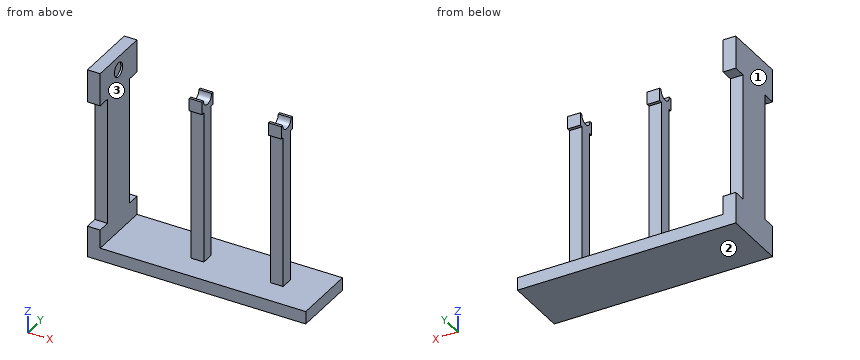
```python
from build123d import *

# Parameters (mm, degrees)
F0_W      = 411.1625
F0_H      = 127
F1_DEPTH  = 25.4
F2_W      = 25.4
F2_H      = 25.4
F3_DEPTH  = 304.8
F4_W      = 25.4
F4_H      = 38.1
F5_DEPTH  = 25.4
F7_DEPTH  = 258.7635
F8_W      = 127
F8_H      = 382.02858
F9_DEPTH  = 25.4
F10_W     = 89.525855
F10_H     = 254
F11_DEPTH = 25.4
F12_R     = 14.2875
F13_DEPTH = 340.36


with BuildPart() as f1:
    # F0 (on Top) → F1 (new body)
    with BuildSketch(Plane.XY):
        with Locations((0, 6.35)):
            Rectangle(F0_W, F0_H)
    extrude(amount=F1_DEPTH)

    # F2 (on face) → F3 (join)
    with BuildSketch(Plane.XY.offset(25.4)):
        with Locations((-40.48125, 6.35)):
            Rectangle(F2_W, F2_H)
        with Locations((118.26875, 6.35)):
            Rectangle(F2_W, F2_H)
    extrude(amount=F3_DEPTH)

    # F4 (on face) → F5 (join)
    with BuildSketch(Plane.XY.offset(330.2)):
        with Locations((-40.48125, 6.35)):
            Rectangle(F4_W, F4_H)
        with Locations((118.26875, 6.35)):
            Rectangle(F4_W, F4_H)
    extrude(amount=F5_DEPTH)

    # F6 (on face) → F7 (cut, through all)
    with BuildSketch(Plane(origin=(-53.18125, 0, 0), x_dir=(0, -1, 0), z_dir=(-1, 0, 0))):
        with BuildLine():
            Line((7.9375, 355.6), (-20.6375, 355.6))
            ThreePointArc((-20.6375, 355.6), (-6.35, 341.3125), (7.9375, 355.6))
        make_face()
    extrude(amount=-F7_DEPTH, mode=Mode.SUBTRACT)

    # F8 (on face) → F9 (join)
    with BuildSketch(Plane(origin=(-205.58125, 0, 0), x_dir=(0, -1, 0), z_dir=(-1, 0, 0))):
        with Locations((-6.35, 191.01429)):
            Rectangle(F8_W, F8_H)
    extrude(amount=F9_DEPTH)

    # F10 (on face) → F11 (cut)
    with BuildSketch(Plane(origin=(-230.98125, 0, 0), x_dir=(0, -1, 0), z_dir=(-1, 0, 0))):
        with Locations((-89.212927, 189.356351)):
            Rectangle(F10_W, F10_H)
        with Locations((76.512927, 189.356351)):
            Rectangle(F10_W, F10_H)
    extrude(amount=-F11_DEPTH, mode=Mode.SUBTRACT)

    # F12 (on face) → F13 (cut)
    with BuildSketch(Plane.YZ.offset(130.96875)):
        with Locations((6.35, 355.6)):
            Circle(F12_R)
    extrude(amount=-F13_DEPTH, mode=Mode.SUBTRACT)


solid = f1.part
```
Input: part model. Units: mm. Frame: model coordinates. Face numbers are marked on the shaded views. Coordinates: 2 decimals unless noted, no trailing zeros. Loops run counter-clockwise (first coordinate to the right, second up) from the corner with the lowest first, then second, coordinate; pieces in that order, holes last. Notation, with made-up numbers: (-6.75, 60.5) -> (2.25, 60.5) arc R19 ccw to (2.25, 75.5) -> close; hole circle Ø2 at (72.25, 29). An arc over 180 degrees is marked (long way). Use a Markdown table: item, result.
1) Cut plane B-B (y = 60). Return the cut outline in (x, z), then the cut area to 3 significant figures.
Results found:
| item | result |
|---|---|
| outline | (-230.98, 0) -> (205.58, 0) -> (205.58, 25.4) -> (-205.58, 25.4) -> (-205.58, 62.36) -> (-230.98, 62.36) -> close; (-230.98, 316.36) -> (-205.58, 316.36) -> (-205.58, 382.03) -> (-230.98, 382.03) -> close |
| area | 13,700 mm2 |
2) Pull-direction query (X, two-part tool) for the marked faces 1, 2 and 3; classes: released by +X, released by -X, zero draft, split by the parting line, or undercut.
Results found:
| item | result |
|---|---|
| face 1 | released by -X |
| face 2 | zero draft |
| face 3 | undercut |
3) Material intervals for line 1 along X through (y, z) = (16, 343); line 2 along Z through (x, y) = (-207.75, 6.35); line 3 along Y through (x, z) = (-207, 355), sorted ascending. Write a range as from..to.
Results found:
| item | result |
|---|---|
| line 1 | x = -230.98..-205.58, -53.18..-27.78, 105.57..130.97 |
| line 2 | z = 0..341.31, 369.89..382.03 |
| line 3 | y = -57.15..-7.92, 20.62..69.85 |
4) Contact query for flat-ended pins moving along their axis: pin 1 (1 mm diameter, centred on x = -154, y = 3, fed in from +Z); pin 2 (1.4 mm diameter, centred on x = 114, y = 24, fed in from +Z); pin 3 (12.5 mm diameter, centred on x = -34, z = 113, fed in from -Y). Output: stop coordinate, or through.
Results found:
| item | result |
|---|---|
| pin 1 | stops at z = 25.4 |
| pin 2 | stops at z = 355.6 |
| pin 3 | stops at y = -6.35 |
5) Cut plane D-D (z = 38). Return the cut outline in (x, y).
Results found:
| item | result |
|---|---|
| outline | (-230.98, -57.15) -> (-205.58, -57.15) -> (-205.58, 69.85) -> (-230.98, 69.85) -> close; (-53.18, -6.35) -> (-27.78, -6.35) -> (-27.78, 19.05) -> (-53.18, 19.05) -> close; (105.57, -6.35) -> (130.97, -6.35) -> (130.97, 19.05) -> (105.57, 19.05) -> close |
6) Cut plane A-A (z = 183.5). Return the cut outline in (x, y), then the cut area to 3 significant figures.
Results found:
| item | result |
|---|---|
| outline | (-230.98, -31.75) -> (-205.58, -31.75) -> (-205.58, 44.45) -> (-230.98, 44.45) -> close; (-53.18, -6.35) -> (-27.78, -6.35) -> (-27.78, 19.05) -> (-53.18, 19.05) -> close; (105.57, -6.35) -> (130.97, -6.35) -> (130.97, 19.05) -> (105.57, 19.05) -> close |
| area | 3,230 mm2 |
